Build history of the part. All positions in model axes, mm. Round coordinates to 2 decimals unless told otherwise and drop trailing zeros. Write each loop counter-clockwise with the first axis right and the second up, starting at its lowest first coordinate (ties: lowest second). Pieces come first, ordered by that corner, then holes.
1) Saw through at D-D (z = 7.5). Write the cut outline in (x, y).
2) Saw through at C-C (x = -90). Write the cut outline in (y, z), plus the area to 4 significant figures.
3) Wall check: probe 1 along X at (y, z) = (2.7, 7.5); probe 2 along X at (y, z) = (2, 60); probe 3 along Z at (x, y) = (-68, 3.2). Give the ranges that are in metal, low to high.
4) Saw through at A-A (x = -7.5). Write the cut outline in (y, z).
5) Saw through at B-B (z = 60). Write the cut outline in (x, y), plus the area to 4 significant figures.
6) Flat gauge pin, fed straight in: pin 1 (3.5 mm diameter, centred on x = -7.5, z = 60, fed in from +Y). Where does the tip first touch, or does it go through?
7) Pull direction Z, two halves, no side cores. Call faces 1 (the cylindrical face through (-7.034, 2.535, 91.478)), 2 (the flat face through (-59, 2, 0)), 3 (the flat face through (-48, 0, 46)): +Z half, -Z half, draft (parallel to the pull), parting line (faces both ways), or undercut.
from build123d import *

# Parameters (mm, degrees)
BOSS_EXTRUDE1_DEPTH = 5
SKETCH3_R           = 1.55
CUT_EXTRUDE1_DEPTH  = 5
SKETCH4_R           = 2.125
CUT_EXTRUDE2_DEPTH  = 5


with BuildPart() as part:
    # Sketch2 → Boss-Extrude1 (new body)
    with BuildSketch(Plane(origin=(0, 0, 0), x_dir=(1, 0, 0), z_dir=(0, 1, 0))):
        Polygon((-120, -15), (-15, -120), (0, -120), (0, 0), (-120, 0), align=None)
    extrude(amount=BOSS_EXTRUDE1_DEPTH)

    # Sketch3 → Cut-Extrude1 (cut)
    with BuildSketch(Plane(origin=(0, 5, 0), x_dir=(1, 0, 0), z_dir=(0, 1, 0))):
        with Locations(Location((-90, -7.5, 0), (0, 0, 270))):
            Circle(SKETCH3_R)
        with Locations(Location((-60, -7.5, 0), (0, 0, 270))):
            Circle(SKETCH3_R)
        with Locations(Location((-7.5, -90, 0), (0, 0, 270))):
            Circle(SKETCH3_R)
        with Locations(Location((-7.5, -60, 0), (0, 0, 270))):
            Circle(SKETCH3_R)
    extrude(amount=-CUT_EXTRUDE1_DEPTH, mode=Mode.SUBTRACT)

    # Sketch4 → Cut-Extrude2 (cut)
    with BuildSketch(Plane(origin=(0, 5, 0), x_dir=(1, 0, 0), z_dir=(0, 1, 0))):
        with Locations(Location((-66.085786438, -37.80151519, 0), (0, 0, 270))):
            Circle(SKETCH4_R)
        with Locations(Location((-73.156854249, -44.872583002, 0), (0, 0, 270))):
            Circle(SKETCH4_R)
        with Locations(Location((-44.872583002, -73.156854249, 0), (0, 0, 90))):
            Circle(SKETCH4_R)
        with Locations(Location((-37.80151519, -66.085786438, 0), (0, 0, 90))):
            Circle(SKETCH4_R)
    extrude(amount=-CUT_EXTRUDE2_DEPTH, mode=Mode.SUBTRACT)


solid = part.part
Evaluation:
1. outline: (-120, 0) - (-91.55, 0) - (-91.55, 5) - (-120, 5) - close; (-88.45, 0) - (-61.55, 0) - (-61.55, 5) - (-88.45, 5) - close; (-58.45, 0) - (0, 0) - (0, 5) - (-58.45, 5) - close
2. outline: (0, 0) - (5, 0) - (5, 5.95) - (0, 5.95) - close; (0, 9.05) - (5, 9.05) - (5, 45) - (0, 45) - close
2. area: 209.5 mm2
3. probe 1: x = -120 to -91.55, -88.45 to -61.55, -58.45 to 0
3. probe 2: x = -75 to -9.05, -5.95 to 0
3. probe 3: z = 0 to 36.88, 38.72 to 67
4. outline: (0, 0) - (5, 0) - (5, 58.45) - (0, 58.45) - close; (0, 61.55) - (5, 61.55) - (5, 88.45) - (0, 88.45) - close; (0, 91.55) - (5, 91.55) - (5, 120) - (0, 120) - close
5. outline: (-75, 0) - (-9.05, 0) - (-9.05, 5) - (-75, 5) - close; (-5.95, 0) - (0, 0) - (0, 5) - (-5.95, 5) - close
5. area: 359.5 mm2
6. pin 1: stops at y = 5
7. face 1: undercut
7. face 2: -Z half
7. face 3: draft
